Print and shaded views of the part. All mm, measured from the part's lowest x, y and z. Round coordinates to 2 decimals unless told otherwise and drop trailing zeros. Loops run counter-clockwise (first coordinate to the right, second up) from the corner with the lowest first, then second, coordinate; pieces in that order, holes last. Notation, with made-up numbers: (-15.5, 21.25) -> (12.5, 21.25) arc R17 ccw to (12.5, 30.25) -> close; hole circle Ø9 at (-25.5, 78). An arc over 180 degrees is marked (long way). Answer as CSV lines item,"result".
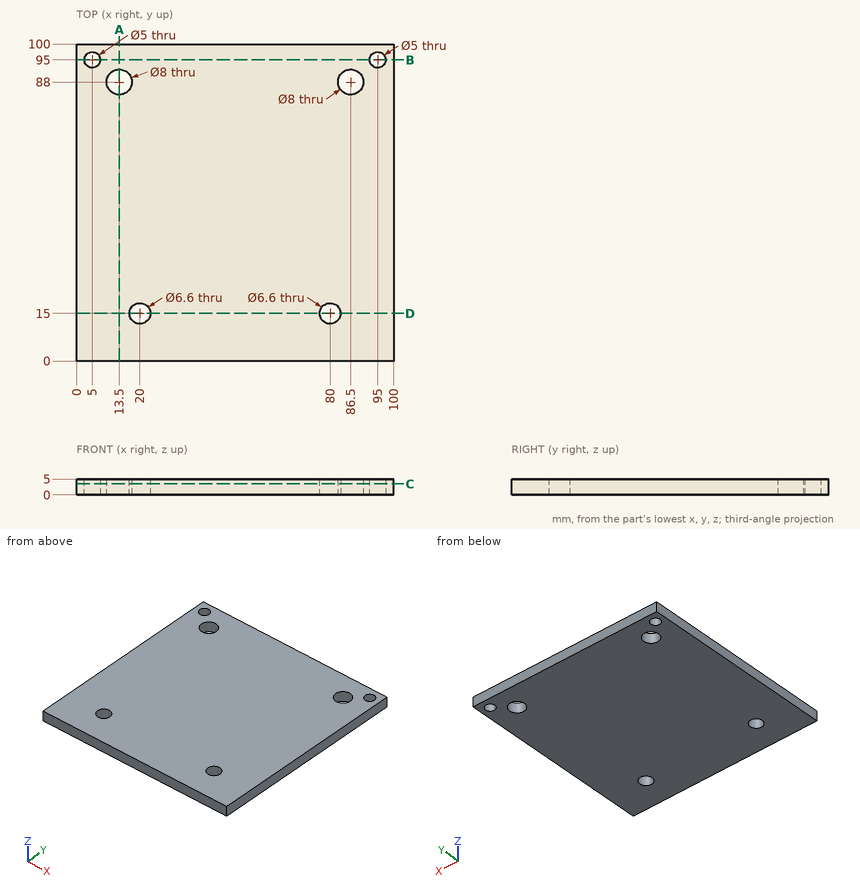
Q1. Drill centre lines: line 1 along Y through (x, z) = (13.5, 2.75); line 2 along Y through (x, z) = (95, 2.7); line 3 along X through (y, z) = (16.5, 0.85). Where is each one in solid material? Low to high.
Geometry results:
line 1,"0 to 84, 92 to 100"
line 2,"0 to 92.5, 97.5 to 100"
line 3,"0 to 17.06, 22.94 to 77.06, 82.94 to 100"
Q2. Saw through at D-D, the plane y = 15. Write the cut outline in (x, z).
Geometry results:
outline,"(0, 0) -> (16.7, 0) -> (16.7, 5) -> (0, 5) -> close; (23.3, 0) -> (76.7, 0) -> (76.7, 5) -> (23.3, 5) -> close; (83.3, 0) -> (100, 0) -> (100, 5) -> (83.3, 5) -> close"
Q3. Saw through at C-C, the plane z = 3.5. Write the cut outline in (x, y), then the cut area to 3 significant figures.
Geometry results:
outline,"(0, 0) -> (100, 0) -> (100, 100) -> (0, 100) -> close; hole circle Ø5 at (5, 95); hole circle Ø8 at (13.5, 88); hole circle Ø6.6 at (20, 15); hole circle Ø6.6 at (80, 15); hole circle Ø8 at (86.5, 88); hole circle Ø5 at (95, 95)"
area,"9,790 mm2"
Q4. Saw through at A-A, the plane x = 13.5. Write the cut outline in (y, z), then the cut area to 3 significant figures.
Geometry results:
outline,"(0, 0) -> (84, 0) -> (84, 5) -> (0, 5) -> close; (92, 0) -> (100, 0) -> (100, 5) -> (92, 5) -> close"
area,"460 mm2"
Q5. Drop flat-ended pins along their axis: P1, Ø6.5, axis at x = 86.5, y = 88, coming from the -Z side; P2, Ø8.5, axis at x = 20, y = 15, coming from the -Z side. Give the stop position or say it passes through.
Geometry results:
P1,"through"
P2,"z = 0"
Q6. Saw through at B-B, the plane y = 95. Write the cut outline in (x, z).
Geometry results:
outline,"(0, 0) -> (2.5, 0) -> (2.5, 5) -> (0, 5) -> close; (7.5, 0) -> (92.5, 0) -> (92.5, 5) -> (7.5, 5) -> close; (97.5, 0) -> (100, 0) -> (100, 5) -> (97.5, 5) -> close"
